Drawing for the job (mm, zero at the part's lowest x, y, z). A direction names the side the tool comes from. Coordinates: 2 decimals unless noted, no trailing zeros. Loops run counter-clockwise (first coordinate to the right, second up) from the corner with the lowest first, then second, coordinate; pieces in that order, holes last. Notation, with made-up numbers: (4, 37) - (25, 37) arc R20 ccw to (25, 49) - close; hole circle Ø3 at (5.5, -21.75). An arc over 180 degrees is marked (long way). Put each result on its own line as item: value.
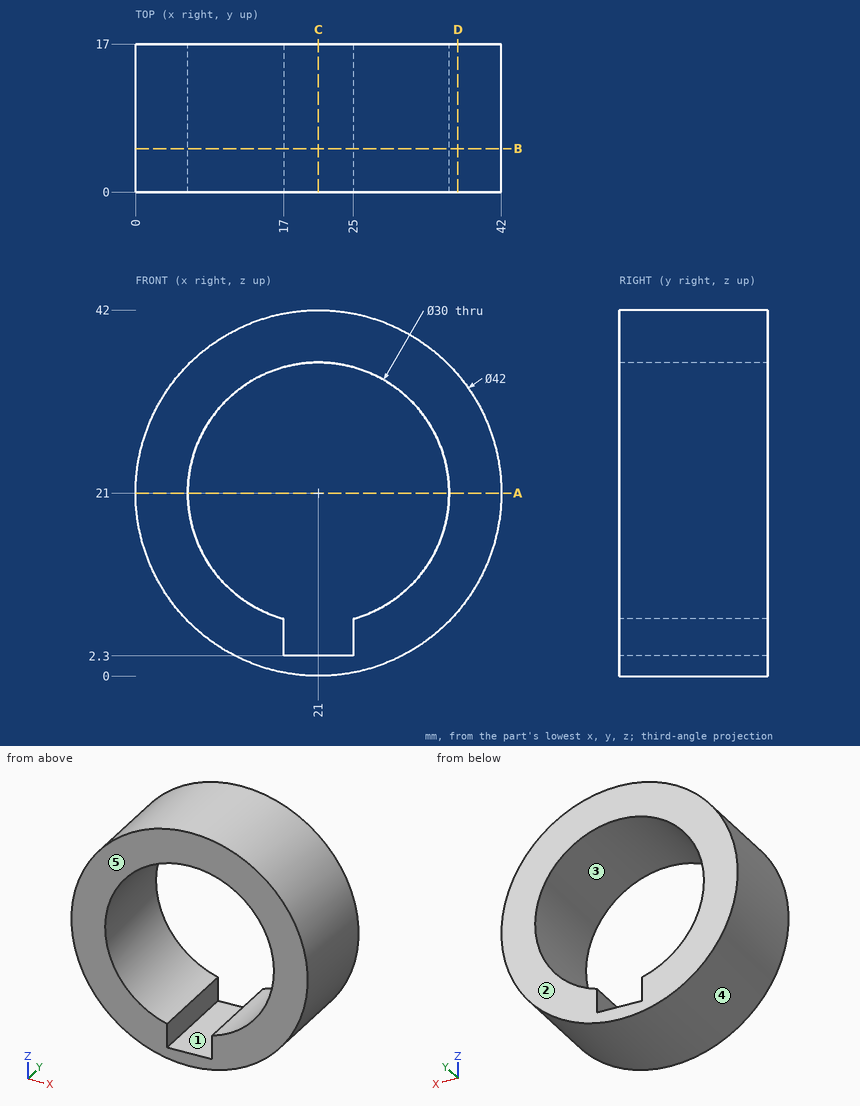
Q1. Tool access for the marked faces 1 and 2: list every direction of +Z, -Z, +X, -X, +Y, -Y with a clear straight run to the whole face (end or side of a thin tool).
Determined:
face 1: +Y, -Y
face 2: +Z, -Z, +X, -X, +Y
Q2. Slice it at D-D, the plane x = 37. Give the cut face in (y, z), then the cut area to 3 significant figures.
Determined:
outline: (0, 7.4) - (17, 7.4) - (17, 34.6) - (0, 34.6) - close
area: 462 mm2
Q3. Wall check: L1, parallel to X at y = 8.25, z = 21; L2, parallel to Z at x = 29, y = 6.5; L3, parallel to Z at x = 32, y = 1. Give the ranges that are in metal, low to high. Write a range as from..to.
Determined:
L1: 0..6, 36..42
L2: 1.58..8.31, 33.69..40.42
L3: 3.11..10.8, 31.2..38.89
Q4. Slice it at A-A, the plane z = 21. Give the cut face in (x, y), then the cut area to 3 significant figures.
Determined:
outline: (0, 0) - (6, 0) - (6, 17) - (0, 17) - close; (36, 0) - (42, 0) - (42, 17) - (36, 17) - close
area: 204 mm2
Q5. Pin check, flat tips, straight feed: pin 1 Ø2 at (y, z) = (5.5, 4) entering from -X; pin 2 Ø9 at (x, y) = (20, 7) entering from +Z; pin 3 Ø8 at (x, y) = (7, 5) entering from +Z; pin 4 Ø4 at (x, y) = (7, 6) entering from +Z. Stop position of each tip, or through.
Determined:
pin 1: x = 7.4
pin 2: z = 42
pin 3: z = 39.47
pin 4: z = 38.23
Q6. Mould opens along X. For the marked faces 3, 4 and 5 say: +X half, -X half, draft (parallel to the pull), parting line (faces both ways), or undercut.
Determined:
face 3: undercut
face 4: parting line
face 5: draft
Q7. Slice it at C-C, the plane x = 21. Give the cut face in (y, z).
Determined:
outline: (0, 0) - (17, 0) - (17, 2.3) - (0, 2.3) - close; (0, 36) - (17, 36) - (17, 42) - (0, 42) - close
Q8. Slice it at B-B, the plane y = 5. Give the cut face in (x, z).
Determined:
outline: circle Ø42 at (21, 21); hole (17, 2.3) - (25, 2.3) - (25, 6.54) arc R15 ccw (long way) to (17, 6.54) - close
